Here's how the part is built. I have some questions about the finished solid (model axes, mm). Round coordinates to 2 decimals unless told otherwise and drop trailing zeros. Loops run counter-clockwise (first coordinate to the right, second up) from the corner with the lowest first, then second, coordinate; pieces in that order, holes last. Notation, with made-up numbers: M 49.25,87.5 L 69.25,87.5 A23 ccw 69.25,118.5 Z; hole C 19.25,-38 d1. An arc over 180 degrees is marked long. Use a Markdown table: item, result.
from build123d import *

# Parameters (mm, degrees)
SKETCH1_W           = 18.3134
SKETCH1_H           = 33
SKETCH1_R           = 0.508
BOSS_EXTRUDE1_DEPTH = 0.425


with BuildPart() as part:
    # Sketch1 → Boss-Extrude1 (new body, symmetric)
    with BuildSketch(Plane(origin=(0, 0, 0), x_dir=(1, 0, 0), z_dir=(0, 1, 0))):
        Rectangle(SKETCH1_W, SKETCH1_H)
        with Locations((-6.35, -15.23)):
            Circle(SKETCH1_R, mode=Mode.SUBTRACT)
        with Locations((-3.81, -15.23)):
            Circle(SKETCH1_R, mode=Mode.SUBTRACT)
        with Locations((-1.27, -15.23)):
            Circle(SKETCH1_R, mode=Mode.SUBTRACT)
        with Locations((1.27, -15.23)):
            Circle(SKETCH1_R, mode=Mode.SUBTRACT)
        with Locations((3.81, -15.23)):
            Circle(SKETCH1_R, mode=Mode.SUBTRACT)
        with Locations((6.35, -15.23)):
            Circle(SKETCH1_R, mode=Mode.SUBTRACT)
        with Locations((-7.366, 15.23)):
            Circle(SKETCH1_R, mode=Mode.SUBTRACT)
        with Locations((-7.366, 12.69)):
            Circle(SKETCH1_R, mode=Mode.SUBTRACT)
        with Locations((-7.366, 10.15)):
            Circle(SKETCH1_R, mode=Mode.SUBTRACT)
        with Locations((-7.366, 7.61)):
            Circle(SKETCH1_R, mode=Mode.SUBTRACT)
        with Locations((-7.366, 5.07)):
            Circle(SKETCH1_R, mode=Mode.SUBTRACT)
        with Locations((-7.366, 2.53)):
            Circle(SKETCH1_R, mode=Mode.SUBTRACT)
        with Locations((-7.366, -0.01)):
            Circle(SKETCH1_R, mode=Mode.SUBTRACT)
        with Locations((-7.366, -2.55)):
            Circle(SKETCH1_R, mode=Mode.SUBTRACT)
        with Locations((-7.366, -5.09)):
            Circle(SKETCH1_R, mode=Mode.SUBTRACT)
        with Locations((-7.366, -7.63)):
            Circle(SKETCH1_R, mode=Mode.SUBTRACT)
        with Locations((-7.366, -10.17)):
            Circle(SKETCH1_R, mode=Mode.SUBTRACT)
        with Locations((-7.366, -12.71)):
            Circle(SKETCH1_R, mode=Mode.SUBTRACT)
        with Locations((7.366, -12.71)):
            Circle(SKETCH1_R, mode=Mode.SUBTRACT)
        with Locations((7.366, -10.17)):
            Circle(SKETCH1_R, mode=Mode.SUBTRACT)
        with Locations((7.366, -7.63)):
            Circle(SKETCH1_R, mode=Mode.SUBTRACT)
        with Locations((7.366, -5.09)):
            Circle(SKETCH1_R, mode=Mode.SUBTRACT)
        with Locations((7.366, -2.55)):
            Circle(SKETCH1_R, mode=Mode.SUBTRACT)
        with Locations((7.366, -0.01)):
            Circle(SKETCH1_R, mode=Mode.SUBTRACT)
        with Locations((7.366, 2.53)):
            Circle(SKETCH1_R, mode=Mode.SUBTRACT)
        with Locations((7.366, 5.07)):
            Circle(SKETCH1_R, mode=Mode.SUBTRACT)
        with Locations((7.366, 7.61)):
            Circle(SKETCH1_R, mode=Mode.SUBTRACT)
        with Locations((7.366, 10.15)):
            Circle(SKETCH1_R, mode=Mode.SUBTRACT)
        with Locations((7.366, 12.69)):
            Circle(SKETCH1_R, mode=Mode.SUBTRACT)
        with Locations((7.366, 15.23)):
            Circle(SKETCH1_R, mode=Mode.SUBTRACT)
    extrude(amount=BOSS_EXTRUDE1_DEPTH, both=True)


solid = part.part
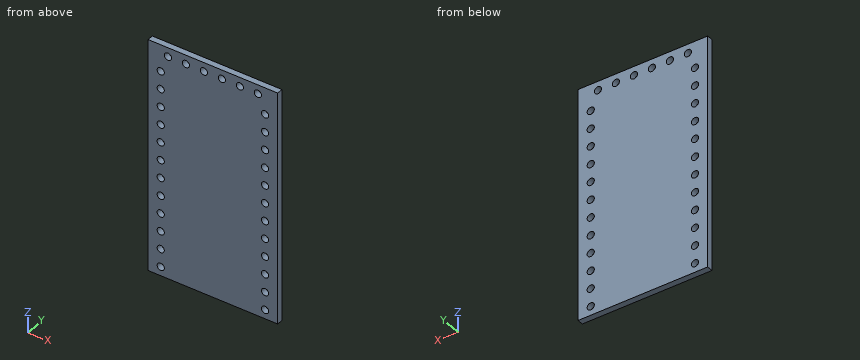
1. Imagine slicing it at D-D, the plane z = 15.23. Write out the boundary of the cut face in (x, y) (3 decimals).
Answer sheet:
| item | result |
|---|---|
| outline | M -9.157,-0.425 L -6.858,-0.425 L -6.858,0.425 L -9.157,0.425 Z; M -5.842,-0.425 L -4.318,-0.425 L -4.318,0.425 L -5.842,0.425 Z; M -3.302,-0.425 L -1.778,-0.425 L -1.778,0.425 L -3.302,0.425 Z; M -0.762,-0.425 L 0.762,-0.425 L 0.762,0.425 L -0.762,0.425 Z; M 1.778,-0.425 L 3.302,-0.425 L 3.302,0.425 L 1.778,0.425 Z; M 4.318,-0.425 L 5.842,-0.425 L 5.842,0.425 L 4.318,0.425 Z; M 6.858,-0.425 L 9.157,-0.425 L 9.157,0.425 L 6.858,0.425 Z |
2. Imagine slicing it at C-C, the plane y = -0.05. State how many separate pieces and enclosed holes the cut face has, then the cut area to 3 significant figures.
Answer sheet:
| item | result |
|---|---|
| separate pieces | 1 |
| enclosed holes | 30 |
| area | 580 mm2 |
3. Imagine slicing it at B-B, the plane x = 1.27. Write out the boundary of the cut face in (y, z) (3 decimals).
Answer sheet:
| item | result |
|---|---|
| outline | M -0.425,-16.5 L 0.425,-16.5 L 0.425,14.722 L -0.425,14.722 Z; M -0.425,15.738 L 0.425,15.738 L 0.425,16.5 L -0.425,16.5 Z |
4. I need wall thicknesses on probe 1 along X at (y, z) = (-0.1, 2.55); probe 2 along Z at (x, y) = (3.75, 0.2); probe 3 along Z at (x, y) = (-1, -0.2). Which ranges of each line are inside material? Lowest first, please. Write a range as from..to.
Answer sheet:
| item | result |
|---|---|
| probe 1 | -9.16..-7.87, -6.86..6.86, 7.87..9.16 |
| probe 2 | -16.5..14.73, 15.73..16.5 |
| probe 3 | -16.5..14.8, 15.66..16.5 |
5. Imagine slicing it at A-A, the plane z = -10.15. Write out the boundary of the cut face in (x, y) (3 decimals).
Answer sheet:
| item | result |
|---|---|
| outline | M -9.157,-0.425 L -7.874,-0.425 L -7.874,0.425 L -9.157,0.425 Z; M -6.858,-0.425 L 6.858,-0.425 L 6.858,0.425 L -6.858,0.425 Z; M 7.874,-0.425 L 9.157,-0.425 L 9.157,0.425 L 7.874,0.425 Z |
